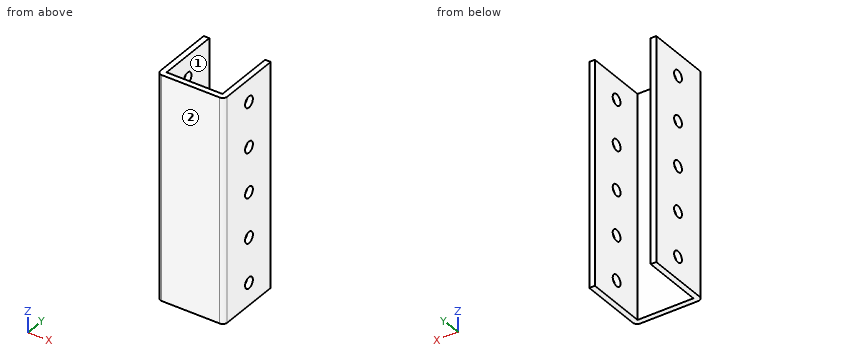
```python
from build123d import *

# Parameters (mm, degrees)
SKETCH2_W           = 38.1
SKETCH2_H           = 127
BOSS_EXTRUDE1_DEPTH = 38.1
SKETCH3_W           = 31.75
SKETCH3_H           = 34.925
CUT_EXTRUDE1_DEPTH  = 406.4
FILLET1_R           = 2.54
SKETCH4_R           = 3.175
CUT_EXTRUDE2_DEPTH  = 50.8


with BuildPart() as part:
    # Sketch2 → Boss-Extrude1 (new body)
    with BuildSketch(Plane(origin=(0, 0, 0), x_dir=(1, 0, 0), z_dir=(0, 1, 0))):
        Rectangle(SKETCH2_W, SKETCH2_H)
    extrude(amount=BOSS_EXTRUDE1_DEPTH)

    # Sketch3 → Cut-Extrude1 (cut)
    with BuildSketch(Plane.XY.offset(63.5)):
        with Locations((0, 20.6375)):
            Rectangle(SKETCH3_W, SKETCH3_H)
    extrude(amount=-CUT_EXTRUDE1_DEPTH, mode=Mode.SUBTRACT)

    # Fillet1
    fillet1_edges = [part.edges().sort_by_distance(p)[0] for p in [
        (-19.05, 0, 0),
        (19.05, 0, 0),
    ]]
    fillet(fillet1_edges, radius=FILLET1_R)

    # Sketch4 → Cut-Extrude2 (cut)
    with BuildSketch(Plane(origin=(19.05, 0, 0), x_dir=(0, 0, -1), z_dir=(1, 0, 0))):
        with Locations((-50.8, 20.32)):
            Circle(SKETCH4_R)
        with Locations((-25.4, 20.32)):
            Circle(SKETCH4_R)
        with Locations((0, 20.32)):
            Circle(SKETCH4_R)
        with Locations((25.4, 20.32)):
            Circle(SKETCH4_R)
        with Locations((50.8, 20.32)):
            Circle(SKETCH4_R)
    extrude(amount=-CUT_EXTRUDE2_DEPTH, mode=Mode.SUBTRACT)


solid = part.part
```
The model under review builds one solid part; all positions refer to its coordinate system, in mm. Face numbers are marked on the shaded views. A direction names the side the tool comes from. Give positions to 0.01 mm unless a question says otherwise; leave off trailing zeros. Write each loop counter-clockwise with the first axis right and the second up, starting at its lowest first coordinate (ties: lowest second). Pieces come first, ordered by that corner, then holes. Notation, with made-up numbers: (80.5, 31.25) - (106.5, 31.25) arc R5 cw to (106.5, 35.25) - close; hole circle Ø4 at (63, -20.5). An arc over 180 degrees is marked (long way). Answer in a Markdown table with one row per item. Add a question column.
1. We need section C-C on z = 10.5. Write out the cut boundary in (x, y) (3 decimals), then the cut area to 3 significant figures.
2. Wall thickness on line 1 along X through (y, z) = (7.5, -35) (3 decimals); line 2 along Y through (x, z) = (9.5, -57) (3 decimals); line 3 along Y through (x, z) = (16.7, -50.8) (3 decimals): over which ranges is each line inside the solid? List them lowest first. Write a range as [from, to].
3. Tool access review of the marked faces 1 and 2: name each direction out of +Z, -Z, +X, -X, +Y, -Y from which nothing blocks a thin tool from reaching the whole face with its end or side.
4. We need section B-B on z = 25.4. Write out the cut boundary in (x, y) (3 decimals), then the cut area to 3 significant figures.
5. We need section D-D on x = 7. Write out the cut boundary in (y, z) (3 decimals).
6. We need section A-A on y = 5. Write out the cut boundary in (x, z) (3 decimals).
7. Insertion check: P1, Ø1, axis at x = -2, z = 31, coming from the +Y side (3 decimals). The pin has a flat end and moves straight along its axis. Give the tip position at first contact, or say it passes through.
Ans:
| question | item | result |
|---|---|---|
| 1 | outline | (-19.05, 2.54) arc R2.54 ccw to (-16.51, 0) - (16.51, 0) arc R2.54 ccw to (19.05, 2.54) - (19.05, 38.1) - (15.875, 38.1) - (15.875, 3.175) - (-15.875, 3.175) - (-15.875, 38.1) - (-19.05, 38.1) - close |
| 1 | area | 340 mm^2 |
| 2 | line 1 | x = [-19.05, -15.875], [15.875, 19.05] |
| 2 | line 2 | y = [0, 3.175] |
| 2 | line 3 | y = [0.007, 17.145], [23.495, 38.1] |
| 3 | face 1 | +Z, -Z, +Y |
| 3 | face 2 | +Z, -Z, +X, -X, -Y |
| 4 | outline | (-19.05, 2.54) arc R2.54 ccw to (-16.51, 0) - (16.51, 0) arc R2.54 ccw to (19.05, 2.54) - (19.05, 17.145) - (15.875, 17.145) - (15.875, 3.175) - (-15.875, 3.175) - (-15.875, 17.145) - (-19.05, 17.145) - close; (-19.05, 23.495) - (-15.875, 23.495) - (-15.875, 38.1) - (-19.05, 38.1) - close; (15.875, 23.495) - (19.05, 23.495) - (19.05, 38.1) - (15.875, 38.1) - close |
| 4 | area | 300 mm^2 |
| 5 | outline | (0, -63.5) - (3.175, -63.5) - (3.175, 63.5) - (0, 63.5) - close |
| 6 | outline | (-19.05, -63.5) - (-15.875, -63.5) - (-15.875, 63.5) - (-19.05, 63.5) - close; (15.875, -63.5) - (19.05, -63.5) - (19.05, 63.5) - (15.875, 63.5) - close |
| 7 | P1 | stops at y = 3.175 |
